Verification items for the finished model (mm, model axes). A direction names the side the tool comes from. Round coordinates to 2 decimals unless told otherwise and drop trailing zeros. Loops run counter-clockwise (first coordinate to the right, second up) from the corner with the lowest first, then second, coordinate; pieces in that order, holes last. Notation, with made-up numbers: (46, 89.25) - (76, 89.25) arc R19 ccw to (76, 103.25) - close; hole circle Ø8 at (8.5, 14). An arc over 180 degrees is marked (long way). Use a Markdown table: item, result. Add a question column.
```python
from build123d import *

# Parameters (mm, degrees)
F0_R     = 11.2
F0_R_2   = 13.2
F1_DEPTH = 7


with BuildPart() as f1:
    # F0 (on Top) → F1 (new body)
    with BuildSketch(Plane.XY):
        with BuildLine():
            ThreePointArc((21.859796, 2.191562), (14.647279, 11.035914), (12.254917, 22.194749))
            ThreePointArc((12.254917, 22.194749), (10.931223, 34.498756), (0, 40.299542))
            ThreePointArc((0, 40.299542), (-10.375988, 35.25913), (-12.827846, 23.987249))
            ThreePointArc((-12.827846, 23.987249), (-12.632849, 20.911303), (-12.827846, 17.835357))
            ThreePointArc((-12.827846, 17.835357), (-16.881022, 7.166958), (-25.348675, -0.484305))
            ThreePointArc((-25.348675, -0.484305), (-35.342411, -7.782661), (-34.900427, -20.149771))
            ThreePointArc((-34.900427, -20.149771), (-25.347308, -26.615434), (-14.359644, -23.102865))
            ThreePointArc((-14.359644, -23.102865), (-11.793295, -21.39602), (-9.03195, -20.026919))
            ThreePointArc((-9.03195, -20.026919), (2.233743, -18.202873), (13.093758, -21.710444))
            ThreePointArc((13.093758, -21.710444), (24.411188, -26.716095), (34.900427, -20.149771))
            ThreePointArc((34.900427, -20.149771), (35.723296, -8.643695), (27.18749, -0.884384))
            ThreePointArc((27.18749, -0.884384), (24.426145, 0.484717), (21.859796, 2.191562))
        make_face()
        with Locations((-23.468892, -13.549771)):
            Circle(F0_R, mode=Mode.SUBTRACT)
        with Locations((23.468892, -13.549771)):
            Circle(F0_R, mode=Mode.SUBTRACT)
        Circle(F0_R_2, mode=Mode.SUBTRACT)
        with Locations((0, 27.099542)):
            Circle(F0_R, mode=Mode.SUBTRACT)
        with BuildLine():
            ThreePointArc((-12.827846, 23.987249), (-10.375988, 35.25913), (0, 40.299542))
            ThreePointArc((0, 40.299542), (-28.341803, 33.676362), (-40.126432, 7.063454))
            ThreePointArc((-40.126432, 7.063454), (-29.025745, 18.908185), (-12.827846, 17.835357))
            ThreePointArc((-12.827846, 17.835357), (-12.632849, 20.911303), (-12.827846, 23.987249))
        make_face()
        with BuildLine():
            ThreePointArc((26.180347, 31.218782), (30.887841, 15.68294), (21.859796, 2.191562))
            ThreePointArc((21.859796, 2.191562), (24.426145, 0.484717), (27.18749, -0.884384))
            ThreePointArc((27.18749, -0.884384), (35.723296, -8.643695), (34.900427, -20.149771))
            ThreePointArc((34.900427, -20.149771), (43.335487, 7.706541), (26.180347, 31.218782))
        make_face()
        with BuildLine():
            ThreePointArc((-14.359644, -23.102865), (-25.347308, -26.615434), (-34.900427, -20.149771))
            ThreePointArc((-34.900427, -20.149771), (-14.993684, -41.382903), (13.946085, -38.282236))
            ThreePointArc((13.946085, -38.282236), (-1.862096, -34.591125), (-9.03195, -20.026919))
            ThreePointArc((-9.03195, -20.026919), (-11.793295, -21.39602), (-14.359644, -23.102865))
        make_face()
    extrude(amount=F1_DEPTH)


solid = f1.part
```
Q1. Thickness scan on line 1 along X through (y, z) = (-10.5, 1); line 2 along Y through (x, z) = (8, 6.25); line 3 along Y through (x, z) = (-21, 1.25). Record the ranges inside material, lowest first.
Q2. Section check A-A on x = -3. Record the cut outline in (y, z).
Q3. Go/stop test with flat-tipped pins: pin 1 Ø2 at (x, z) = (8, 1) entering from -Y; pin 2 Ø1 at (y, z) = (-26, 2) entering from +X; pin 3 Ø6 at (x, y) = (-29, 18) entering from -Z. Record where each tip stops, or that it passes through.
Q4. Set-up check for faces 5 (the face through (14.72, 10.89, 3.45)), 6 (the face through (-35.26, -7.62, 3.45)): record each of +Z, -Z, +X, -X, +Y, -Y from which the full face is reachable in a straight line by a thin tool's end or side.
Q5. Section check B-B on y = -23.5. Record the cut outline in (x, z), plus the area to 3 significant figures.
Q6. Section check D-D on z = 3.5. Record the cut outline in (x, y), plus the area to 3 significant figures.
Q7. Section check C-C on x = -32. Record the cut outline in (y, z), plus the area to 3 significant figures.
Q8. Release check for a two-part mould opening along X. For faces 1 (the face through (11.03, 34.35, 3.45)), 2 (the face through (-1.677, -34.736, 3.451)), 3 (the face through (-15.389, -41.233, 3.451)), 4 (the face through (43.4, 7.3, 3.5)) record: +X half, -X half, draft (parallel to the pull), parting line (faces both ways), or undercut.
Determined:
| question | item | result |
|---|---|---|
| 1 | line 1 | x = -36.31 to -34.25, -12.69 to -8, 8 to 12.69, 34.25 to 41.2 |
| 1 | line 2 | y = -41.28 to -38.61, -19.35 to -10.5, 10.5 to 19.26, 34.94 to 37.6 |
| 1 | line 3 | y = -38.42 to -24.47, -2.63 to 2.54, 20.2 to 38.27 |
| 2 | outline | (-43.42, 0) - (-33.61, 0) - (-33.61, 7) - (-43.42, 7) - close; (-18.37, 0) - (-12.85, 0) - (-12.85, 7) - (-18.37, 7) - close; (12.85, 0) - (16.31, 0) - (16.31, 7) - (12.85, 7) - close; (37.89, 0) - (40.86, 0) - (40.86, 7) - (37.89, 7) - close |
| 3 | pin 1 | stops at y = -41.64 |
| 3 | pin 2 | stops at x = 29.08 |
| 3 | pin 3 | stops at z = 0 |
| 4 | face 5 | +Z, -Z |
| 4 | face 6 | +Z, -Z, -X |
| 5 | outline | (-33.69, 0) - (-28.61, 0) - (-28.61, 7) - (-33.69, 7) - close; (-18.33, 0) - (-8.66, 0) - (-8.66, 7) - (-18.33, 7) - close; (14.8, 0) - (18.33, 0) - (18.33, 7) - (14.8, 7) - close; (28.61, 0) - (32.14, 0) - (32.14, 7) - (28.61, 7) - close |
| 5 | area | 153 mm² |
| 6 | outline | (-40.13, 7.06) arc R18.98 cw to (-12.83, 17.84) arc R24.36 cw to (-25.35, -0.48) arc R13.2 ccw to (-34.9, -20.15) arc R32.64 ccw to (13.95, -38.28) arc R18.98 cw to (-9.03, -20.03) arc R24.36 cw to (13.09, -21.71) arc R13.2 ccw to (34.9, -20.15) arc R32.64 ccw to (26.18, 31.22) arc R18.98 cw to (21.86, 2.19) arc R24.36 cw to (12.25, 22.19) arc R13.2 ccw to (0, 40.3) arc R32.64 ccw to start; hole circle Ø22.4 at (-23.47, -13.55); hole circle Ø26.4 at (0, 0); hole circle Ø22.4 at (0, 27.1); hole circle Ø22.4 at (23.47, -13.55) |
| 6 | area | 2,330 mm² |
| 7 | outline | (-26.93, 0) - (-20.81, 0) - (-20.81, 7) - (-26.93, 7) - close; (-6.29, 0) - (-3.48, 0) - (-3.48, 7) - (-6.29, 7) - close; (17.42, 0) - (30.13, 0) - (30.13, 7) - (17.42, 7) - close |
| 7 | area | 152 mm² |
| 8 | face 1 | undercut |
| 8 | face 2 | undercut |
| 8 | face 3 | parting line |
| 8 | face 4 | +X half |
